```python
from build123d import *

# Parameters (mm, degrees)
SKETCH1_R                    = 50
BOSS_EXTRUDE1_DEPTH          = 5
F_10_2_10_2_DIAMETER_HOLE1_D = 10.2
M3_CLEARANCE_HOLE1_D         = 3.4
SKETCH12_R                   = 12.5
CUT_EXTRUDE2_DEPTH           = 10
SKETCH13_R                   = 2
CUT_EXTRUDE3_DEPTH           = 10
CIRPATTERN1_COUNT            = 4
SKETCH14_R                   = 4
CUT_EXTRUDE4_DEPTH           = 10
SKETCH15_R                   = 7.5
CUT_EXTRUDE5_DEPTH           = 10


with BuildPart() as part:
    # Sketch1 → Boss-Extrude1 (new body)
    with BuildSketch(Plane.XY):
        Circle(SKETCH1_R)
    extrude(amount=BOSS_EXTRUDE1_DEPTH)

    # Ø10.2 (10.2) Diameter Hole1 (through all)
    with Locations(Plane(origin=(0, 0, 0), x_dir=(-1, 0, 0), z_dir=(0, 0, -1))):
        with Locations((37, 0), (-37, 0), (0, -40)):
            Hole(F_10_2_10_2_DIAMETER_HOLE1_D / 2)

    # M3 Clearance Hole1 (through all)
    with Locations(Plane.XY.offset(5)):
        with Locations((46, 0), (28, 0), (9, -40), (-9, -40), (-46, 0), (-28, 0)):
            Hole(M3_CLEARANCE_HOLE1_D / 2)

    # Sketch12 → Cut-Extrude2 (cut)
    with BuildSketch(Plane.XY.offset(5)):
        with Locations((0, 26)):
            Circle(SKETCH12_R)
    extrude(amount=-CUT_EXTRUDE2_DEPTH, mode=Mode.SUBTRACT)

    # Sketch13 → Cut-Extrude3 (cut)
    with BuildSketch(Plane.XY.offset(5)):
        with Locations((-15.5, 41.5)):
            Circle(SKETCH13_R)
    cut_extrude3 = extrude(amount=-CUT_EXTRUDE3_DEPTH, mode=Mode.SUBTRACT)

    # CirPattern1: Cut-Extrude3 ×4 about axis
    cirpattern1_axis = Axis((0, 26, 0), (0, 0, 1))
    for i in range(1, CIRPATTERN1_COUNT):
        add(cut_extrude3.rotate(cirpattern1_axis, i * 360 / CIRPATTERN1_COUNT), mode=Mode.SUBTRACT)

    # Sketch14 → Cut-Extrude4 (cut)
    with BuildSketch(Plane.XY.offset(5)):
        with Locations((-39.87754263, -18.595203517)):
            Circle(SKETCH14_R)
        with Locations((39.87754263, -18.595203517)):
            Circle(SKETCH14_R)
    extrude(amount=-CUT_EXTRUDE4_DEPTH, mode=Mode.SUBTRACT)

    # Sketch15 → Cut-Extrude5 (cut)
    with BuildSketch(Plane.XY.offset(5)):
        Circle(SKETCH15_R)
    extrude(amount=-CUT_EXTRUDE5_DEPTH, mode=Mode.SUBTRACT)


solid = part.part
```
Geometry: final body of the model. Coordinates: model frame, mm. Coordinates: 2 decimals unless noted, no trailing zeros. Loops run counter-clockwise (first coordinate to the right, second up) from the corner with the lowest first, then second, coordinate; pieces in that order, holes last. Notation, with made-up numbers: M -24.75,-1 L -5.75,-1 A22 ccw -5.75,27 Z; hole C -14.75,55 d10. An arc over 180 degrees is marked long. Put each result on its own line as item: value.
(1) Cut plane A-A on y = 0. State how many separate pieces and enclosed holes the cut face has, then the cut area to 3 significant figures.
Answer sheet:
separate pieces: 8
enclosed holes: 0
area: 255 mm^2
(2) Draft query along Y for faces 1 (the face through (47.69, 15.02, 2.46)), 2 (the face through (-1, -10, 5)), 3 (the face through (15.76, 8.517, 2.535)). Return one class per face: pulls with the +Y half, pulls with the -Y half, needs draft (parallel to the pull), parting line crosses it, or undercut.
Answer sheet:
face 1: parting line crosses it
face 2: needs draft
face 3: undercut
(3) Cut plane B-B on x = -9. Return the cut outline in (y, z).
Answer sheet:
outline: M -49.18,0 L -41.7,0 L -41.7,5 L -49.18,5 Z; M -38.3,0 L 17.33,0 L 17.33,5 L -38.3,5 Z; M 34.67,0 L 49.18,0 L 49.18,5 L 34.67,5 Z
(4) Cut plane D-D on x = 28. Return the cut outline in (y, z).
Answer sheet:
outline: M -41.42,0 L -1.7,0 L -1.7,5 L -41.42,5 Z; M 1.7,0 L 41.42,0 L 41.42,5 L 1.7,5 Z
(5) Material intervals for probe 1 along Y at (x, z) = (0, 2.45); probe 2 along X at (y, z) = (-18, 3.3); probe 3 along Y at (x, z) = (-6, 0.5), sorted ascending.
Answer sheet:
probe 1: y = -50 to -45.1, -34.9 to -7.5, 7.5 to 13.5, 38.5 to 50
probe 2: x = -46.65 to -43.83, -35.92 to 35.92, 43.83 to 46.65
probe 3: y = -49.64 to -4.5, 4.5 to 15.03, 36.97 to 49.64
(6) First-contact query: pin 1 (2 mm diameter, centred on y = -16, z = 1, fed in from +X); pin 2 (1.5 mm diameter, centred on y = -39, z = 1, fed in from -X). Flat tips, straight axial feed; report the tip coordinate or a pass-through.
Answer sheet:
pin 1: stops at x = 47.7
pin 2: stops at x = -32.2
